from build123d import *

# Parameters (mm, degrees)
FORMSENKUNG_F_R_M2_LINSENSENKSCHRAUBE_MI_D           = 2.4
FORMSENKUNG_F_R_M2_LINSENSENKSCHRAUBE_MI_DEPTH       = 5
FORMSENKUNG_F_R_M2_LINSENSENKSCHRAUBE_MI_CSINK_D     = 4.4
FORMSENKUNG_F_R_M2_LINSENSENKSCHRAUBE_MI_CSINK_ANGLE = 90
FORMSENKUNG_F_R_M2_LINSENSENKSCHRAUBE_MI_TIP         = 0.721032743


with BuildPart() as part:
    # Skizze1 → Rotation1 (revolve)
    with BuildSketch(Plane.XY):
        with BuildLine():
            Line((0, 0), (0, 4))
            Line((0, 4), (-0.499279021, 4))
            ThreePointArc((-0.499279021, 4), (-1.000662513, 3.498616507), (-1.502046006, 4))
            Line((-1.502046006, 4), (-2, 4))
            Line((-2, 4), (-2, 0))
            Line((-2, 0), (0, 0))
        make_face()
    revolve(axis=Axis((0, 0, 0), (-1, 0, 0)))

    # Formsenkung für M2 Linsensenkschraube mit Schlitz1
    with Locations(Plane.ZY.offset(2)):
        with Locations((0, 0)):
            CounterSinkHole(FORMSENKUNG_F_R_M2_LINSENSENKSCHRAUBE_MI_D / 2, FORMSENKUNG_F_R_M2_LINSENSENKSCHRAUBE_MI_CSINK_D / 2, depth=FORMSENKUNG_F_R_M2_LINSENSENKSCHRAUBE_MI_DEPTH, counter_sink_angle=FORMSENKUNG_F_R_M2_LINSENSENKSCHRAUBE_MI_CSINK_ANGLE)
            with Locations((0, 0, -(FORMSENKUNG_F_R_M2_LINSENSENKSCHRAUBE_MI_DEPTH + FORMSENKUNG_F_R_M2_LINSENSENKSCHRAUBE_MI_TIP / 2))):  # 118° drill point
                Cone(0, FORMSENKUNG_F_R_M2_LINSENSENKSCHRAUBE_MI_D / 2, FORMSENKUNG_F_R_M2_LINSENSENKSCHRAUBE_MI_TIP, mode=Mode.SUBTRACT)


solid = part.part
Can you work these out from the model? Positions are in its coordinate system, mm. Give positions to 0.01 mm unless a question says otherwise; leave off trailing zeros. Loops run counter-clockwise (first coordinate to the right, second up) from the corner with the lowest first, then second, coordinate; pieces in that order, holes last. Notation, with made-up numbers: (65.25, -10) - (74.25, -10) arc R27 cw to (74.25, 16) - close; hole circle Ø3 at (33.25, -15.75). An arc over 180 degrees is marked (long way). Return JSON: item names as keys, results as strings.
1. I'm going to push flat-ended pins straight in: pin 1 Ø1 at (x, z) = (-0.5, 3) entering from -Y; pin 2 Ø1.9 at (y, z) = (0, 0) entering from +X; pin 3 Ø1 at (x, z) = (-0.5, 2.5) entering from +Y. Where does each tip first touch, or does it pass through?
Output values:
{"pin 1": "stops at y = -3.12", "pin 2": "passes through", "pin 3": "stops at y = 3.46"}
2. If I drill on line 1 (Y direction, x = -0.45, z = 0); line 2 (Y direction, x = -0.65, z = 0); line 3 (X direction, y = 2.75, z = 2.5), over which ranges is the centre line in solid material (lowest first)?
Output values:
{"line 1": "y = -4 to -1.2, 1.2 to 4", "line 2": "y = -3.64 to -1.2, 1.2 to 3.64", "line 3": "x = -2 to -1.41, -0.59 to 0"}
3. I want a section at C-C on x = -1.85. Please give me the cut outline in (y, z), and give its area (3 significant figures).
Output values:
{"outline": "circle Ø8 at (0, 0); hole circle Ø4.1 at (0, 0)", "area": "37.1 mm²"}
4. We'd pull the mould along Y, two halves only. Please class faces 1 (the face through (-0.49, 1.01, -0.65)), 2 (the face through (-1.755, -0.867, 3.905)), 3 (the face through (0, 1, 1)): +Y half, -Y half, draft (parallel to the pull), parting line (faces both ways), or undercut.
Output values:
{"face 1": "undercut", "face 2": "parting line", "face 3": "draft"}
5. I want a section at D-D on x = -1.4. Please give me the cut outline in (y, z).
Output values:
{"outline": "circle Ø7.39 at (0, 0); hole circle Ø3.2 at (0, 0)"}
6. I want a section at A-A on z = 0. Please give me the cut outline in (x, y).
Output values:
{"outline": "(-2, -4) - (-1.5, -4) arc R0.5 cw to (-0.5, -4) - (0, -4) - (0, -1.2) - (-1, -1.2) - (-2, -2.2) - close; (-2, 2.2) - (-1, 1.2) - (0, 1.2) - (0, 4) - (-0.5, 4) arc R0.5 cw to (-1.5, 4) - (-2, 4) - close"}
